Verification items for the finished model (mm, model axes). Face numbers are marked on the shaded views. A direction names the side the tool comes from. Give positions to 0.01 mm unless a question says otherwise; leave off trailing zeros. Write each loop counter-clockwise with the first axis right and the second up, starting at its lowest first coordinate (ties: lowest second). Pieces come first, ordered by that corner, then holes. Notation, with made-up numbers: (14.25, 33.25) -> (30.25, 33.25) arc R29 cw to (30.25, 64.25) -> close; hole circle Ø2 at (-32, -18.5). An arc over 180 degrees is marked (long way). Answer as CSV lines item,"result". Start each with the question number.
1) Material ranges on L1, parallel to Z at x = 13.5, y = 7.5; L2, parallel to Z at x = -4, y = 3.5; L3, parallel to Z at x = 14, y = 13, recorded low to high.
2) Tool access check on the marked faces 1 and 2. Record the directions out of +Z, -Z, +X, -X, +Y, -Y that give a thin tool (end or side, any length) a straight path to the whole face; none if there is none.
3) Sectioned sample at C-C on z = 281.5. Record the cut outline in (x, y), and give its area (3 significant figures).
4) Sectioned sample at D-D on z = 209.5. Record the cut outline in (x, y).
5) Gauge pin test, flat ends, axial feed: pin 1 Ø3 at (x, y) = (5.5, -17.5) entering from -Z; pin 2 Ø1.5 at (y, z) = (-10.5, 222.5) entering from +X; pin 3 Ø1.5 at (x, z) = (10.5, 96.5) entering from +Y. Record the tip position at first contact, or that the pin passes through.
6) Sectioned sample at B-B on y = 0. Record the cut outline in (x, z), and give its area (3 significant figures).
7) Sectioned sample at A-A on x = 0. Record the cut outline in (y, z), and give its area (3 significant figures).
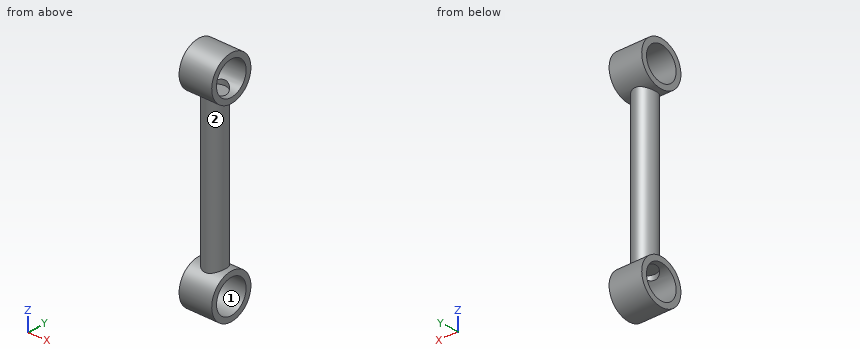
```python
from build123d import *

# Parameters (mm, degrees)
SKETCH4_R           = 25.4
SKETCH4_R_2         = 19.177
BOSS_EXTRUDE3_DEPTH = 19.05
SKETCH6_R           = 12.7
BOSS_EXTRUDE4_DEPTH = 203.2
CUT_EXTRUDE2_START  = -12.7
SKETCH8_R           = 12.7
CUT_EXTRUDE2_DEPTH  = 12.7
SKETCH9_R           = 12.7
CUT_EXTRUDE4_DEPTH  = 12.7


with BuildPart() as part:
    # Sketch4 → Boss-Extrude3 (new, symmetric)
    with BuildSketch(Plane(origin=(0, 0, 0), x_dir=(0, 0, -1), z_dir=(1, 0, 0))):
        with Locations(Location((-284.396079729, 0, 0), (0, 0, 180))):
            Circle(SKETCH4_R)
        with Locations(Location((-284.396079729, 0, 0), (0, 0, 180))):
            Circle(SKETCH4_R_2, mode=Mode.SUBTRACT)
    boss_extrude3 = extrude(amount=BOSS_EXTRUDE3_DEPTH, both=True)

    # Sketch6 → Boss-Extrude4 (add)
    with BuildSketch(Plane.XY.offset(276.86)):
        Circle(SKETCH6_R)
    extrude(amount=-BOSS_EXTRUDE4_DEPTH)

    # Mirror1: Boss-Extrude3 across plane
    add(boss_extrude3.mirror(Plane(origin=(0, 0, 175.26), x_dir=(1, 0, 0), z_dir=(0, 0, -1))))

    # Sketch8 → Cut-Extrude2 (cut)
    with BuildSketch(Plane(origin=(0, 0, 73.66), x_dir=(-1, 0, 0), z_dir=(0, 0, -1)).offset(CUT_EXTRUDE2_START)):
        with Locations(Location((0, 0, 0), (0, 0, 180))):
            Circle(SKETCH8_R)
    extrude(amount=CUT_EXTRUDE2_DEPTH, mode=Mode.SUBTRACT)

    # Sketch9 → Cut-Extrude4 (cut)
    with BuildSketch(Plane.XY.offset(276.86)):
        Circle(SKETCH9_R)
    extrude(amount=-CUT_EXTRUDE4_DEPTH, mode=Mode.SUBTRACT)


solid = part.part
```
Ans:
1,L1,"z = 41.86 to 48.47, 83.77 to 90.39, 260.13 to 266.75, 302.05 to 308.66"
1,L2,"z = 40.97 to 47.27, 86.36 to 264.16, 303.25 to 309.55"
1,L3,"z = 44.3 to 52.03, 80.22 to 87.95, 262.57 to 270.3, 298.49 to 306.22"
2,face 1,"+X, -X"
2,face 2,"none"
3,outline,"(-19.05, -25.23) -> (19.05, -25.23) -> (19.05, -18.96) -> (-19.05, -18.96) -> close; (-19.05, 18.96) -> (19.05, 18.96) -> (19.05, 25.23) -> (-19.05, 25.23) -> close"
3,area,"478 mm²"
4,outline,"circle Ø25.4 at (0, 0)"
5,pin 1,"stops at z = 46.4"
5,pin 2,"stops at x = 8.14"
5,pin 3,"stops at y = 8.14"
6,outline,"(-19.05, 40.72) -> (19.05, 40.72) -> (19.05, 46.95) -> (-19.05, 46.95) -> close; (-19.05, 85.3) -> (-12.7, 85.3) -> (-12.7, 86.36) -> (12.7, 86.36) -> (12.7, 85.3) -> (19.05, 85.3) -> (19.05, 91.52) -> (12.7, 91.52) -> (12.7, 259) -> (19.05, 259) -> (19.05, 265.22) -> (12.7, 265.22) -> (12.7, 264.16) -> (-12.7, 264.16) -> (-12.7, 265.22) -> (-19.05, 265.22) -> (-19.05, 259) -> (-12.7, 259) -> (-12.7, 91.52) -> (-19.05, 91.52) -> close; (-19.05, 303.57) -> (19.05, 303.57) -> (19.05, 309.8) -> (-19.05, 309.8) -> close"
6,area,"5,150 mm²"
7,outline,"(-12.7, 88.12) arc R25.4 ccw (long way) to (12.7, 88.12) -> (12.7, 262.4) arc R25.4 ccw (long way) to (-12.7, 262.4) -> close; hole (-12.7, 80.49) arc R19.18 ccw (long way) to (12.7, 80.49) -> (12.7, 86.36) -> (-12.7, 86.36) -> close; hole (-12.7, 264.16) -> (12.7, 264.16) -> (12.7, 270.03) arc R19.18 ccw (long way) to (-12.7, 270.03) -> close"
7,area,"5,920 mm²"
